```python
from build123d import *

# Parameters (mm, degrees)
SKETCH2_W           = 37
SKETCH2_H           = 37
BOSS_EXTRUDE1_DEPTH = 15
SKETCH3_W           = 29
SKETCH3_H           = 29
CUT_EXTRUDE1_DEPTH  = 12
SKETCH4_R           = 4
CUT_EXTRUDE2_DEPTH  = 12
BOSS_EXTRUDE3_START = 12
SKETCH5_R           = 4
BOSS_EXTRUDE3_DEPTH = 12
SKETCH6_R           = 3
CUT_EXTRUDE3_DEPTH  = 12
FILLET3_R           = 1
FILLET4_R           = 1
FILLET6_R           = 0.5


with BuildPart() as part:
    # Sketch2 → Boss-Extrude1 (new body)
    with BuildSketch(Plane.XY):
        Rectangle(SKETCH2_W, SKETCH2_H)
    extrude(amount=BOSS_EXTRUDE1_DEPTH)

    # Sketch3 → Cut-Extrude1 (cut)
    with BuildSketch(Plane.XY.offset(15)):
        Rectangle(SKETCH3_W, SKETCH3_H)
    extrude(amount=-CUT_EXTRUDE1_DEPTH, mode=Mode.SUBTRACT)

    # Sketch4 → Cut-Extrude2 (cut)
    with BuildSketch(Plane(origin=(0, 0, 0), x_dir=(-1, 0, 0), z_dir=(0, 0, -1))):
        Circle(SKETCH4_R)
    extrude(amount=-CUT_EXTRUDE2_DEPTH, mode=Mode.SUBTRACT)

    # Sketch5 → Boss-Extrude3 (add)
    with BuildSketch(Plane(origin=(0, 0, 1), x_dir=(-1, 0, 0), z_dir=(0, 0, -1)).offset(BOSS_EXTRUDE3_START)):
        Circle(SKETCH5_R)
    extrude(amount=-BOSS_EXTRUDE3_DEPTH)

    # Sketch6 → Cut-Extrude3 (cut)
    with BuildSketch(Plane(origin=(0, 0, -11), x_dir=(-1, 0, 0), z_dir=(0, 0, -1))):
        Circle(SKETCH6_R)
    extrude(amount=-CUT_EXTRUDE3_DEPTH, mode=Mode.SUBTRACT)

    # Fillet3
    fillet3_edges = [part.edges().sort_by_distance(p)[0] for p in [
        (4, 0, 0),
        (0, 18.5, 0),
        (18.5, 0, 0),
        (0, -18.5, 0),
        (-18.5, 0, 0),
    ]]
    fillet(fillet3_edges, radius=FILLET3_R)

    # Fillet4
    fillet4_edges = [part.edges().sort_by_distance(p)[0] for p in [
        (-14.5, 0, 3),
        (0, 14.5, 3),
        (14.5, 0, 3),
        (0, -14.5, 3),
        (4, 0, 3),
    ]]
    fillet(fillet4_edges, radius=FILLET4_R)

    # Fillet6
    fillet6_edges = [part.edges().sort_by_distance(p)[0] for p in [
        (4, 0, 1),
        (3, 0, 1),
    ]]
    fillet(fillet6_edges, radius=FILLET6_R - 0.0001)  # a hair under: the kernel refuses the full size


solid = part.part
```
Check sheet for the modelled part. Datum: model origin and axes. Units: mm. A direction names the side the tool comes from. Round coordinates to 2 decimals unless told otherwise and drop trailing zeros. Order: outer loops, then holes, each group sorted by start corner. A loop starts at its lowest first (then second) coordinate and runs counter-clockwise, first axis right, second up. Notation, with made-up numbers: (40.25, -7) - (91.25, -7) arc R32 cw to (91.25, 28) - close; hole circle Ø9 at (3, -10.75). An arc over 180 degrees is marked (long way). Answer as CSV lines item,"result". Start each with the question number.
1) Section check D-D (y = 15.5). Record the cut outline in (x, z), then the cut area to 3 significant figures.
2) Scan lines: probe 1 along X at (y, z) = (-0.5, 4.25); probe 2 along Y at (x, z) = (0, -2.25); probe 3 along Y at (x, z) = (0, 1.85). Record each from-to range of solid material in increasing order.
3) Tool access check on faces 1 (the face through (-14.5, 0, 10)), 2 (the face through (0.867, -3.905, -6.07)), 3 (the face through (18.199, 0.259, 0.285)). Record the directions out of +Z, -Z, +X, -X, +Y, -Y that give a thin tool (end or side, any length) a straight path to the whole face; none if there is none.
4) Draft check along Y on faces 4 (the face through (0.259, -18.199, 0.285)), 5 (the face through (-1, 3, -11)), 6 (the face through (0, -14.5, 10)). Enter one of: +Y half, -Y half, draft (parallel to the pull), parting line (faces both ways), or undercut.
5) Depth check by flat-ended pin: pin 1 (12 mm diameter, centred on y = -9, z = -7.5, fed in from -X); pin 2 (7 mm diameter, centred on x = 0, y = 0, fed in from -Z); pin 3 (8 mm diameter, centred on x = 6, y = -2, fed in from +Z); pin 4 (5.5 mm diameter, centred on x = -1.5, y = 0, fed in from +Z). Enter the tip coordinate at first touch or a pass-through.
6) Section check C-C (z = 8.5). Record the cut outline in (x, y), then the cut area to 3 significant figures.
Determined:
1,outline,"(-18.5, 1) arc R1 ccw to (-17.5, 0) - (17.5, 0) arc R1 ccw to (18.5, 1) - (18.5, 15) - (-18.5, 15) - close"
1,area,"555 mm^2"
2,probe 1,"-18.5 to -14.5, 14.5 to 18.5"
2,probe 2,"-4 to -3, 3 to 4"
2,probe 3,"-18.5 to -4, 4 to 18.5"
3,face 1,"+Z"
3,face 2,"-Z"
3,face 3,"-Z, +X, +Y, -Y"
4,face 4,"-Y half"
4,face 5,"draft"
4,face 6,"undercut"
5,pin 1,"x = -2.65"
5,pin 2,"z = -11"
5,pin 3,"z = 3"
5,pin 4,"z = 2.66"
6,outline,"(-18.5, -18.5) - (18.5, -18.5) - (18.5, 18.5) - (-18.5, 18.5) - close; hole (-14.5, -14.5) - (14.5, -14.5) - (14.5, 14.5) - (-14.5, 14.5) - close"
6,area,"528 mm^2"
